Source: CAD feature listing. Evaluate the final solid. Frame: model axes, mm. A direction names the side the tool comes from. Give positions to 0.01 mm unless a question says otherwise; leave off trailing zeros. Order: outer loops, then holes, each group sorted by start corner. A loop starts at its lowest first (then second) coordinate and runs counter-clockwise, first axis right, second up. Notation, with made-up numbers: (-16, -22) -> (1, -22) arc R5 cw to (1, -16) -> close; hole circle Ø11 at (10, -39.75). An arc over 180 degrees is marked (long way). Use CSV: the item, a comma, the result in double quotes.
```python
from build123d import *

# Parameters (mm, degrees)
SKETCH1_R           = 2
BOSS_EXTRUDE1_DEPTH = 1.6
SKETCH2_R           = 1
BOSS_EXTRUDE2_DEPTH = 10
FILLET1_R           = 0.5
CUT_EXTRUDE1_DEPTH  = 0.55


with BuildPart() as part:
    # Sketch1 → Boss-Extrude1 (new body)
    with BuildSketch(Plane(origin=(0, 0, 0), x_dir=(1, 0, 0), z_dir=(0, 1, 0))):
        with Locations(Location((0, 0, 0), (0, 0, 270))):
            Circle(SKETCH1_R)
    extrude(amount=BOSS_EXTRUDE1_DEPTH)

    # Sketch2 → Boss-Extrude2 (add)
    with BuildSketch(Plane.XZ):
        with Locations(Location((0, 0, 0), (0, 0, 90))):
            Circle(SKETCH2_R)
    extrude(amount=BOSS_EXTRUDE2_DEPTH)

    # Fillet1
    fillet1_edges = [part.edges().sort_by_distance(p)[0] for p in [
        (0, 1.6, -2),
    ]]
    fillet(fillet1_edges, radius=FILLET1_R)

    # Sketch3 → Cut-Extrude1 (cut)
    with BuildSketch(Plane(origin=(0, 1.6, 0), x_dir=(1, 0, 0), z_dir=(0, 1, 0))):
        Polygon((-2, -0.25), (-0.25, -0.25), (-0.25, -2), (0.25, -2), (0.25, -0.25), (2, -0.25), (2, 0.25), (0.25, 0.25), (0.25, 2), (-0.06766133, 2.298366751), (-0.25, 2), (-0.25, 0.25), (-2, 0.25), align=None)
    extrude(amount=-CUT_EXTRUDE1_DEPTH, mode=Mode.SUBTRACT)


solid = part.part
```
1. Access query for faces 1 (the flat face through (0, -10, 0)), 2 (the flat face through (-1, 0, 1)). Directions: +Z, -Z, +X, -X, +Y, -Y. A direction counts if a zero-diameter tool reaches every point of the face in a straight line with its end or side. Return the directions, or none.
Answer below:
face 1,"+Z, -Z, +X, -X, -Y"
face 2,"-Y"
2. Ray query, line 1 along Y through (x, z) = (0.6, -1.15); line 2 along X through (y, z) = (1.25, -1.45); line 3 along Y through (x, z) = (0.2, -1.7). Return the intervals inside material, ascending.
Answer below:
line 1,"y = 0 to 1.6"
line 2,"x = -1.34 to -0.25, 0.25 to 1.34"
line 3,"y = 0 to 1.05"
3. Mould query, pull axis X, two halves, no side actions, for faces 3 (the cylindrical face through (1, -5, 0)), 4 (the flat face through (0, 1.05, 0)), 5 (the flat face through (0.7, 1.6, 0.7)). Classes: released by +X, released by -X, zero draft, split by the parting line, or undercut.
Answer below:
face 3,"split by the parting line"
face 4,"undercut"
face 5,"zero draft"
4. Section query A-A on z = 0. Return loops of the section in (x, y), plus the area to 3 significant figures.
Answer below:
outline,"(-2, 0) -> (-1, 0) -> (-1, -10) -> (1, -10) -> (1, 0) -> (2, 0) -> (2, 1.05) -> (-2, 1.05) -> close"
area,"24.2 mm²"
5. Section query B-B on x = 0. Return loops of the section in (y, z).
Answer below:
outline,"(-10, -1) -> (0, -1) -> (0, -2) -> (1.05, -2) -> (1.05, 2) -> (0, 2) -> (0, 1) -> (-10, 1) -> close"
6. Section query C-C on y = -6.25. Return loops of the section in (x, z).
Answer below:
outline,"circle Ø2 at (0, 0)"
7. Pin query (flat end, axial travel): P1, Ø0.6, axis at x = -1.5, y = 1.5, coming from the -Z side; P2, Ø0.6, axis at y = 1.5, z = -1.5, coming from the -X side; P3, Ø1, axis at x = 0.5, y = -7, coming from the +Z side. Return the tip coordinate at first contact, or that it passes through.
Answer below:
P1,"stops at z = -1.49"
P2,"stops at x = -1.49"
P3,"stops at z = 1"
